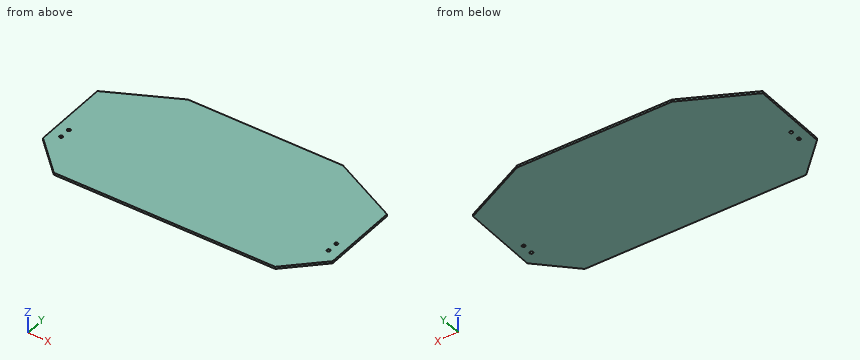
from build123d import *

# Parameters (mm, degrees)
SKETCH_1_R      = 1.5
EXTRUDE_1_DEPTH = 2


with BuildPart() as part:
    # 草图1 → 凸台-拉伸1 (new body)
    with BuildSketch(Plane.XY):
        Polygon((-130.81475452, 0), (-130.81475452, 70), (-70, 100), (70, 100), (130.81475452, 70), (130.81475452, 0), (100, -30), (-100, -30), align=None)
        with Locations((-120.81475452, 9)):
            Circle(SKETCH_1_R, mode=Mode.SUBTRACT)
        with Locations(Location((120.81475452, 9, 0), (0, 0, 180))):
            Circle(SKETCH_1_R, mode=Mode.SUBTRACT)
        with Locations((-120.81475452, 19)):
            Circle(SKETCH_1_R, mode=Mode.SUBTRACT)
        with Locations(Location((120.81475452, 19, 0), (0, 0, 180))):
            Circle(SKETCH_1_R, mode=Mode.SUBTRACT)
    extrude(amount=EXTRUDE_1_DEPTH)


solid = part.part
Input: part model. Units: mm. Frame: model coordinates. Coordinates: 2 decimals unless noted, no trailing zeros. Loops run counter-clockwise (first coordinate to the right, second up) from the corner with the lowest first, then second, coordinate; pieces in that order, holes last.
Q1. Cut plane B-B (y = 80). Output: boundary loops of the cut face in (x, z).
Q2. Material intervals for line 1 (Y direction, x = -96, z = 1.2); line 2 (X direction, y = 71, z = 1.6); line 3 (Y direction, x = -113, z = 0.3), sorted ascending.
Q3. Contact query for a flat-ended pin moving along its axis: pin 1 (4 mm diameter, centred on x = -120.81, y = 19, fed in from +Z). Output: stop coordinate, or through.
Q4. Cut plane A-A (z = 1.4). Output: boundary loops of the cut face in (x, y).
Q5. Cut plane C-C (y = -9). Output: boundary loops of the cut face in (x, z).
Working result:
1. outline: (-110.54, 0) - (110.54, 0) - (110.54, 2) - (-110.54, 2) - close
2. line 1: y = -30 to 87.17
2. line 2: x = -128.79 to 128.79
2. line 3: y = -17.34 to 78.79
3. pin 1: stops at z = 2
4. outline: (-130.81, 0) - (-100, -30) - (100, -30) - (130.81, 0) - (130.81, 70) - (70, 100) - (-70, 100) - (-130.81, 70) - close; hole circle Ø3 at (-120.81, 9); hole circle Ø3 at (-120.81, 19); hole circle Ø3 at (120.81, 9); hole circle Ø3 at (120.81, 19)
5. outline: (-121.57, 0) - (121.57, 0) - (121.57, 2) - (-121.57, 2) - close
